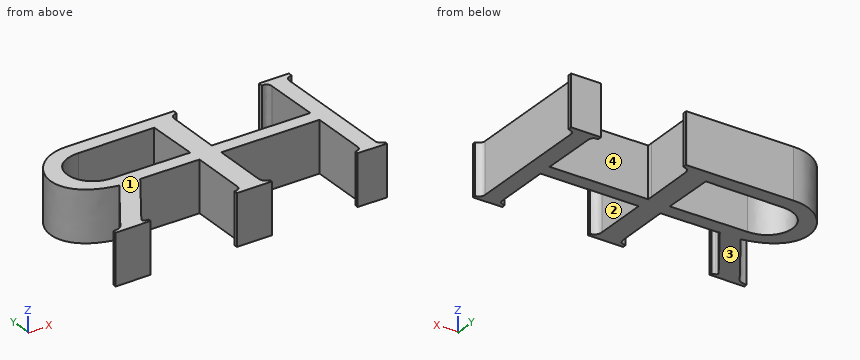
```python
from build123d import *

# Parameters (mm, degrees)
F1_DEPTH = 3


# Not quite as in the source:
# - ends of sketch curves that miss each other by under 0.0002 mm in the source are joined


with BuildPart() as f1:
    # F0 (on Top) → F1 (new body)
    with BuildSketch(Plane.XY):
        with BuildLine():
            Line((1.1892447866, 4.276448), (-5.1239697534, 4.2621811105))
            add(Edge.make_bspline(
                [(-5.1239697534, 4.2621811105), (-7.7808246997, 4.2757478261), (-9.2426975653, 0.2504639081), (-5.1792210147, -0.4118392886)],
                knots=[0, 0, 0, 0, 1, 1, 1, 1], degree=3))
            Line((-5.1792210147, -0.4118392886), (-7.4358199708, -3.8138012247))
            add(Edge.make_bspline(
                [(-7.4358199708, -3.8138012247), (-7.5115597505, -3.9074856806), (-7.537762832, -4.0076449282), (-8.0121770072, -4.0492147307)],
                knots=[0, 0, 0, 0, 1, 1, 1, 1], degree=3))
            Line((-8.0121770072, -4.0492147307), (-8.0121770072, -4.2521576986))
            Line((-8.0121770072, -4.2521576986), (-5.9340439579, -4.2278042412))
            Line((-5.9340439579, -4.2278042412), (-5.9340439579, -4.0654502213))
            add(Edge.make_bspline(
                [(-5.9340439579, -4.0654502213), (-6.0599730098, -4.054522155), (-6.1436827864, -4.0293012572), (-6.1809375378, -4.0026613543)],
                knots=[0, 0, 0, 0, 1, 1, 1, 1], degree=3))
            add(Edge.make_bspline(
                [(-6.1809375378, -4.0026613543), (-6.2530914835, -3.9629456061), (-6.2541383485, -3.9018136478), (-6.2019284451, -3.8219191915)],
                knots=[0, 0, 0, 0, 1, 1, 1, 1], degree=3))
            Line((-6.2019284451, -3.8219191915), (-3.9695588998, -0.4449526542))
            Line((-3.9695588998, -0.4449526542), (-0.4708268475, -0.453070178))
            Line((-0.4708268475, -0.453070178), (-0.4789443713, -3.7001536766))
            add(Edge.make_bspline(
                [(-0.4789443713, -3.7001536766), (-0.4894063767, -3.8582816931), (-0.511182765, -4.0522109002), (-0.8767118972, -4.0573326976)],
                knots=[0, 0, 0, 0, 1, 1, 1, 1], degree=3))
            Line((-0.8767118972, -4.0573326976), (-0.8767118972, -4.276510713))
            Line((-0.8767118972, -4.276510713), (1.2014211521, -4.2683931892))
            Line((1.2014211521, -4.2683931892), (1.2009267376, -4.1117789848))
            add(Edge.make_bspline(
                [(1.2009267376, -4.1117789848), (0.9540548658, -4.0521630537), (0.8074211, -3.9109443668), (0.8117693779, -3.643329238)],
                knots=[0, 0, 0, 0, 1, 1, 1, 1], degree=3))
            Line((0.8117693779, -3.643329238), (0.8117693779, -0.4504044473))
            Line((0.8117693779, -0.4504044473), (6.6162368382, -0.4383405203))
            Line((6.6162368382, -0.4383405203), (6.623033018, -3.7082712004))
            add(Edge.make_bspline(
                [(6.623033018, -3.7082712004), (6.6159065383, -3.8428631383), (6.6131664366, -4.0230470912), (6.2638249484, -4.0654502213)],
                knots=[0, 0, 0, 0, 1, 1, 1, 1], degree=3))
            Line((6.2638249484, -4.0654502213), (6.2587514407, -4.2683931892))
            Line((6.2587514407, -4.2683931892), (7.9878229928, -4.276510713))
            Line((7.9878229928, -4.276510713), (7.9878229928, -4.1060387263))
            add(Edge.make_bspline(
                [(7.9878229928, -4.1060387263), (7.7941463093, -4.0440123031), (7.6495123525, -3.9453779431), (7.6468790194, -3.7407417386)],
                knots=[0, 0, 0, 0, 1, 1, 1, 1], degree=3))
            Line((7.6468790194, -3.7407417386), (7.6225260051, 3.6139009438))
            add(Edge.make_bspline(
                [(7.6225260051, 3.6139009438), (7.6218814055, 3.8627278793), (7.729467946, 4.0122785134), (8.0040584834, 4.0164664167)],
                knots=[0, 0, 0, 0, 1, 1, 1, 1], degree=3))
            Line((8.0040584834, 4.0164664167), (8.0121760072, 4.2633179094))
            Line((8.0121760072, 4.2633179094), (6.2343979833, 4.2551999426))
            Line((6.2343979833, 4.2551999426), (6.2363273516, 4.008799005))
            add(Edge.make_bspline(
                [(6.2363273516, 4.008799005), (6.3452247993, 4.0058905543), (6.6002611554, 4.0485187405), (6.6097418632, 3.6759729985)],
                knots=[0, 0, 0, 0, 1, 1, 1, 1], degree=3))
            Line((6.6097418632, 3.6759729985), (6.6321672813, 0.5291723511))
            Line((6.6321672813, 0.5291723511), (6.6332519216, 0.3769724351))
            Line((6.6332519216, 0.3769724351), (0.8123838086, 0.3769724351))
            Line((0.8123838086, 0.3769724351), (0.8123838086, 0.6393006265))
            Line((0.8123838086, 0.6393006265), (0.8280061975, 3.6544898918))
            add(Edge.make_bspline(
                [(0.8280061975, 3.6544898918), (0.8551715265, 3.8458646241), (0.9207173302, 4.0128832408), (1.2257741664, 4.0279044033)],
                knots=[0, 0, 0, 0, 1, 1, 1, 1], degree=3))
            Line((1.2257741664, 4.0279044033), (1.2328771659, 4.2765093839))
            Line((1.2328771659, 4.2765093839), (1.2099382837, 4.2765100827))
            Line((1.2099382837, 4.2765100827), (1.1892447866, 4.276448))
        make_face()
        with BuildLine():
            Line((-0.456683315, 0.3769724351), (-5.024860472, 0.3920733419))
            add(Edge.make_bspline(
                [(-5.024860472, 0.3920733419), (-7.1084099294, 0.3583060733), (-7.3152098618, 3.3560575894), (-5.0022086687, 3.4048052624)],
                knots=[0, 0, 0, 0, 1, 1, 1, 1], degree=3))
            Line((-5.0022086687, 3.4048052624), (-0.4944369111, 3.450109312))
            Line((-0.4944369111, 3.450109312), (-0.456683315, 0.3769724351))
        make_face(mode=Mode.SUBTRACT)
    extrude(amount=F1_DEPTH)


solid = f1.part
```
For this review, take the finished solid that the model builds, in its own axes (mm). Face numbers are marked on the shaded views. A direction names the side the tool comes from. Coordinates: 2 decimals unless noted, no trailing zeros. Loops run counter-clockwise (first coordinate to the right, second up) from the corner with the lowest first, then second, coordinate; pieces in that order, holes last. Notation, with made-up numbers: (44, -4.5) -> (81, -4.5) arc R16 ccw to (81, 15.5) -> close; hole circle Ø11 at (45.5, -5.5). An arc over 180 degrees is marked (long way). Return JSON: item names as keys, results as strings. Group by question number.
(1) Consider section B-B, the plane y = -1. Give the boundary of the cut face in (x, z).
(2) Consider section D-D, the plane x = 1.5. Give the boundary of the cut face in (y, z).
(3) Consider section A-A, the plane x = -3. Give the boundary of the cut face in (y, z), plus the area to 3 significant figures.
(4) Tool access review of the marked faces 3 and 4: name each direction out of +Z, -Z, +X, -X, +Y, -Y from which nothing blocks a thin tool from reaching the whole face with its end or side.
(5) Consider section C-C, the plane y = -3. Give the boundary of the cut face in (x, z), plus the area to 3 significant figures.
(6) For pin 1 Ø0.9 at (y, z) = (-2, 1.5) entering from +X; pin 2 Ø1.5 at (x, z) = (2, 1.5) entering from -Y; pin 3 Ø1 at (x, z) = (-1.5, 0.5) entering from +Y, all flat-tipped, find the tip position at first contact; note any pin that passes through.
(7) To check wall thickness, follow L1, parallel to X at y = -3.25, z = 2.5; L2, parallel to Y at x = -6.5, z = 2.85; L3, parallel to Y at x = 0.5, z = 2.4. State the ranges of each line that lie inside material, in increasing order.
(8) Mouldability with a two-part tool opening along Y and no side actions: class the marked faces 1 and 2 as pulls with the +Y half, pulls with the -Y half, needs draft (parallel to the pull), parting line crosses it, or undercut.
Results below:
{
 "1": {"outline": "(-5.57, 0) -> (-4.34, 0) -> (-4.34, 3) -> (-5.57, 3) -> close; (-0.47, 0) -> (0.81, 0) -> (0.81, 3) -> (-0.47, 3) -> close; (6.62, 0) -> (7.64, 0) -> (7.64, 3) -> (6.62, 3) -> close"},
 "2": {"outline": "(-0.45, 0) -> (0.38, 0) -> (0.38, 3) -> (-0.45, 3) -> close"},
 "3": {"outline": "(-0.45, 0) -> (0.39, 0) -> (0.39, 3) -> (-0.45, 3) -> close; (3.42, 0) -> (4.27, 0) -> (4.27, 3) -> (3.42, 3) -> close", "area": "5.02 mm2"},
 "4": {"face 3": "-Z, +X, -X, +Y, -Y", "face 4": "+Z, -Z"},
 "5": {"outline": "(-6.9, 0) -> (-5.66, 0) -> (-5.66, 3) -> (-6.9, 3) -> close; (-0.48, 0) -> (0.81, 0) -> (0.81, 3) -> (-0.48, 3) -> close; (6.62, 0) -> (7.64, 0) -> (7.64, 3) -> (6.62, 3) -> close", "area": "10.6 mm2"},
 "6": {"pin 1": "stops at x = 7.64", "pin 2": "stops at y = -0.45", "pin 3": "stops at y = 4.27"},
 "7": {"L1": "x = -7.06 to -5.82, -0.48 to 0.81, 6.62 to 7.65", "L2": "y = -4.23 to -2.4, 0 to 1.22, 2.59 to 3.87", "L3": "y = -4.27 to 4.27"},
 "8": {"face 1": "needs draft", "face 2": "undercut"}
}
